Can you work these out from the model? Positions are in its coordinate system, mm. A direction names the side the tool comes from. Give positions to 0.01 mm unless a question says otherwise; leave off trailing zeros. Loops run counter-clockwise (first coordinate to the right, second up) from the corner with the lowest first, then second, coordinate; pieces in that order, holes last. Notation, with made-up numbers: M -29.75,56 L -8.75,56 A24 ccw -8.75,72 Z; hole C -17,58.5 d8. An arc over 180 degrees is marked long. One line per item, written item: value. Start each with the question number.
Autodesk Inventor part; units mm, degrees
ref_plane "YZ Plane" through (0, 0, 0) normal (1, 0, 0) x (0, 1, 0)
ref_plane "XZ Plane" through (0, 0, 0) normal (0, 1, 0) x (-1, 0, 0)
ref_plane "XY Plane" through (0, 0, 0) normal (0, 0, 1) x (1, 0, 0)
ref_plane "Work Plane1" through (0, 0, 0) normal (0, 0, 1) x (1, 0, 0)
sketch "Sketch1" plane through (0, 0, 0) normal (0, 0, 1) x (1, 0, 0)
  circle A0 centre (0, 0) radius 18.669
  line L0 (13.462, -27.1587) -> (-13.462, -27.1587)
  line L1 (-13.462, -27.1587) -> (-13.462, -12.9347)
  line L2 (-13.462, -12.9347) -> (13.462, -12.9347)
  line L3 (13.462, -12.9347) -> (13.462, -27.1587)
  dimension "d0" = 37.338
  dimension "d1" = 26.924
  dimension "d2" = 14.224
extrude "Extrusion1" add sketch "Sketch1" along normal blind 15.24
sketch "Sketch2" plane through (0, 0, 15.24) normal (0, 0, 1) x (1, 0, 0)
  line L0 (-13.462, -12.9347) -> (-13.462, -27.1587)
  line L1 (-13.462, -27.1587) -> (13.462, -27.1587)
  line L2 (13.462, -27.1587) -> (13.462, -12.9347)
  arc A0 (13.462, -12.9347) -> (-13.462, -12.9347) centre (0, 0) ccw
  circle A1 centre (0, 0) radius 20.066
  dimension "d5" = 40.132
extrude "Extrusion2" add sketch "Sketch2" along normal blind 11.684
sketch "Sketch3" plane through (0, 0, 26.924) normal (0, 0, 1) x (1, 0, 0)
  circle A0 centre (0, 0) radius 20.066
extrude "Extrusion3" add sketch "Sketch3" along normal blind 25.4
sketch "Sketch4" plane through (0, 0, 52.324) normal (0, 0, 1) x (1, 0, 0)
  circle A0 centre (0, 0) radius 20.066
  circle A1 centre (0, 0) radius 17.7904
extrude "Extrusion4" cut sketch "Sketch4" against normal blind 20.32 contours A1
properties part number "dragonFlyLens" material "ABS Plastic"
Q1. For P1, Ø1.5, axis at x = -13.5, z = 10.5, coming from the +Y side; P2, Ø4.5, axis at y = -20, z = 8.5, coming from the +X side; P3, Ø8, axis at x = 1, z = 17, coming from the +Y side, each with a flat end and sliding along its axis, tell me the tip position at first contact or that it passes through.
Q2. If we section it at C-C, the plane z = 20.5: Write out the boundary of the cut face in (x, y), plus the area to 3 significant figures.
Q3. If we section it at A-A, the plane y = 0: Write out the boundary of the cut face in (x, z), plus the area to 3 significant figures.
Q4. If we mould it in two halves opening along X, with no side actions, what happens to faces 1 (the face through (0, -27.159, 13)), 2 (the face through (9.564, 15.001, 42.306)), 3 (the face through (13.462, -20, 13))? For each: released by +X, released by -X, zero draft, split by the parting line, or undercut.
Q5. Which directions (+Z, -Z, +X, -X, +Y, -Y) give clear straight access to the entire face, cutting with the end or side of a thin tool? Please do faces 4 (the face through (-2, -18, 52.324)), 5 (the face through (0, 0, 32.004)), 6 (the face through (-0.61, 18.66, 7.51)).
Q6. If we section it at B-B, the plane x = 0: Write out the boundary of the cut face in (y, z).
Q7. I need wall thicknesses on line 1 along Y through (x, z) = (0, 46); line 2 along X through (y, z) = (-13.5, 8); line 3 along Z through (x, y) = (7, 8.5). Which ranges of each line are inside material? Lowest first, please.
Response:
1. P1: y = 13.64
1. P2: x = 13.46
1. P3: y = 20.07
2. outline: M -13.46,-27.16 L 13.46,-27.16 L 13.46,-14.88 A20.07 ccw long -13.46,-14.88 Z
2. area: 1,500 mm^2
3. outline: M -20.07,15.24 L -18.67,15.24 L -18.67,0 L 18.67,0 L 18.67,15.24 L 20.07,15.24 L 20.07,52.32 L 17.79,52.32 L 17.79,32 L -17.79,32 L -17.79,52.32 L -20.07,52.32 Z
3. area: 1,330 mm^2
4. face 1: zero draft
4. face 2: undercut
4. face 3: released by +X
5. face 4: +Z, +X, -X, +Y, -Y
5. face 5: +Z
5. face 6: -Z
6. outline: M -27.16,0 L 18.67,0 L 18.67,15.24 L 20.07,15.24 L 20.07,52.32 L 17.79,52.32 L 17.79,32 L -17.79,32 L -17.79,52.32 L -20.07,52.32 L -20.07,26.92 L -27.16,26.92 Z
7. line 1: -20.07 to -17.79, 17.79 to 20.07
7. line 2: -13.46 to 13.46
7. line 3: 0 to 32
